```python
from build123d import *

# Parameters (mm, degrees)
F0_W     = 1676.4
F0_H     = 50.8
F1_DEPTH = 50.8
F2_W     = 50.8
F2_H     = 50.8
F3_DEPTH = 50.8
F5_DEPTH = 50.8
F6_W     = 25.4
F6_H     = 15.24
F7_DEPTH = 50.8
F8_W     = 25.4
F8_H     = 15.24
F9_DEPTH = 50.8


with BuildPart() as f1:
    # F0 (on Top) → F1 (new body)
    with BuildSketch(Plane.XY):
        Rectangle(F0_W, F0_H)
    extrude(amount=F1_DEPTH)

    # F2 (on face) → F3 (cut)
    with BuildSketch(Plane(origin=(-838.2, 0, 0), x_dir=(0, -1, 0), z_dir=(-1, 0, 0))):
        with Locations((0, 25.4)):
            Rectangle(F2_W, F2_H)
        Polygon((-12.177117, 33.02), (0, 33.02), (13.222883, 33.02), (13.222883, 17.78), (-12.177117, 17.78), align=None, mode=Mode.SUBTRACT)
    extrude(amount=-F3_DEPTH, mode=Mode.SUBTRACT)

    # F4 (on face) → F5 (cut)
    with BuildSketch(Plane.YZ.offset(838.2)):
        Polygon((25.4, 50.8), (0, 50.8), (-25.4, 50.8), (-25.4, 0), (25.4, 0), align=None)
        Polygon((-12.179509, 33.02), (0, 33.02), (13.220491, 33.02), (13.220491, 17.78), (-12.179509, 17.78), align=None, mode=Mode.SUBTRACT)
    extrude(amount=-F5_DEPTH, mode=Mode.SUBTRACT)

    # F6 (on face) → F7 (cut)
    with BuildSketch(Plane.XZ.offset(25.4)):
        with Locations((-317.5, 25.4)):
            Rectangle(F6_W, F6_H)
    extrude(amount=-F7_DEPTH, mode=Mode.SUBTRACT)

    # F8 (on face) → F9 (cut)
    with BuildSketch(Plane.XZ.offset(25.4)):
        with Locations((114.3, 25.4)):
            Rectangle(F8_W, F8_H)
    extrude(amount=-F9_DEPTH, mode=Mode.SUBTRACT)


solid = f1.part
```
The listing builds one solid part. Answer for the finished solid, in the listing's coordinates (mm). A direction names the side the tool comes from. Round coordinates to 2 decimals unless told otherwise and drop trailing zeros.
Q1. For a pull along Z with two mould halves and no side action, classify faces 5 (the face through (-318, 0, 33.02)), 6 (the face through (-11, 0, 0)), 7 (the face through (114, 0, 33.02)), 8 (the face through (-787.4, 0, 14)) as released by +Z, released by -Z, zero draft, split by the parting line, or undercut.
Q2. Which of the six approach directions +Z, -Z, +X, -X, +Y, -Y give full straight-line access (tool end or side, diameter ignored) to faces 1 (the face through (813, 1, 17.78)), 2 (the face through (-813, -1, 17.78)), 3 (the face through (-318, 0, 17.78)), 4 (the face through (-813, 0, 33.02))?
Q3. Find the intervals of material crossed by line 1 (X direction, y = -15, z = 25); line 2 (X direction, y = 6.5, z = 25); line 3 (X direction, y = -10, z = 11), in increasing order.
Q4. Given pin 1 Ø12.5 at (x, y) = (-800.5, -2.5) entering from +Z; pin 2 Ø12 at (x, z) = (-819.5, 24.5) entering from -Y; pin 3 Ø4.5 at (x, z) = (815, 23.5) entering from -Y, each flat-ended and moving along its own axis, determine where each tip first touches the part or whether it passes through.
Completed:
1. face 5: undercut
1. face 6: released by -Z
1. face 7: undercut
1. face 8: zero draft
2. face 1: -Z, +X, +Y, -Y
2. face 2: -Z, -X, +Y, -Y
2. face 3: +Y, -Y
2. face 4: +Z, -X, +Y, -Y
3. line 1: x = -787.4 to -330.2, -304.8 to 101.6, 127 to 787.4
3. line 2: x = -838.2 to -330.2, -304.8 to 101.6, 127 to 838.2
3. line 3: x = -787.4 to 787.4
4. pin 1: stops at z = 33.02
4. pin 2: stops at y = -13.22
4. pin 3: stops at y = -12.18
